```python
from build123d import *

# Parameters (mm, degrees)
SKETCH1_R                = 22
BOSS_EXTRUDE1_DEPTH      = 2.3
BOSS_EXTRUDE2_DEPTH      = 5
BOSS_EXTRUDE2_DEPTH_BACK = 21.4
SKETCH2_R                = 10.85
SKETCH3_R                = 3.9
BOSS_EXTRUDE3_DEPTH      = 9
SKETCH4_R                = 2.6
CUT_EXTRUDE1_DEPTH       = 38.761885546


with BuildPart() as part:
    # Sketch1 → Boss-Extrude1 (new body)
    with BuildSketch(Plane(origin=(0, 0, 0), x_dir=(1, 0, 0), z_dir=(0, 1, 0))):
        with Locations(Location((0, 0, 0), (0, 0, 270))):
            Circle(SKETCH1_R)
    extrude(amount=BOSS_EXTRUDE1_DEPTH)

    # Sketch2 → Boss-Extrude2 (add, two sides: drawn at the far end of the back side and taken through both)
    with BuildSketch(Plane(origin=(0, 2.3, 0), x_dir=(1, 0, 0), z_dir=(0, 1, 0)).offset(-BOSS_EXTRUDE2_DEPTH_BACK)):
        with Locations(Location((0, 0, 0), (0, 0, 270))):
            Circle(SKETCH2_R)
    extrude(amount=BOSS_EXTRUDE2_DEPTH + BOSS_EXTRUDE2_DEPTH_BACK)

    # Sketch3 → Boss-Extrude3 (add)
    with BuildSketch(Plane(origin=(0, 7.3, 0), x_dir=(1, 0, 0), z_dir=(0, 1, 0))):
        with Locations(Location((0, 0, 0), (0, 0, 270))):
            Circle(SKETCH3_R)
    extrude(amount=BOSS_EXTRUDE3_DEPTH)

    # Sketch4 → Cut-Extrude1 (cut, through all)
    with BuildSketch(Plane(origin=(0, 2.3, 0), x_dir=(1, 0, 0), z_dir=(0, 1, 0))):
        with Locations(Location((0, 17.45, 0), (0, 0, 270))):
            Circle(SKETCH4_R)
        with Locations(Location((-15.112143296, -8.725, 0), (0, 0, 270))):
            Circle(SKETCH4_R)
        with Locations(Location((15.112143296, -8.725, 0), (0, 0, 270))):
            Circle(SKETCH4_R)
    extrude(amount=-CUT_EXTRUDE1_DEPTH, mode=Mode.SUBTRACT)


solid = part.part
```
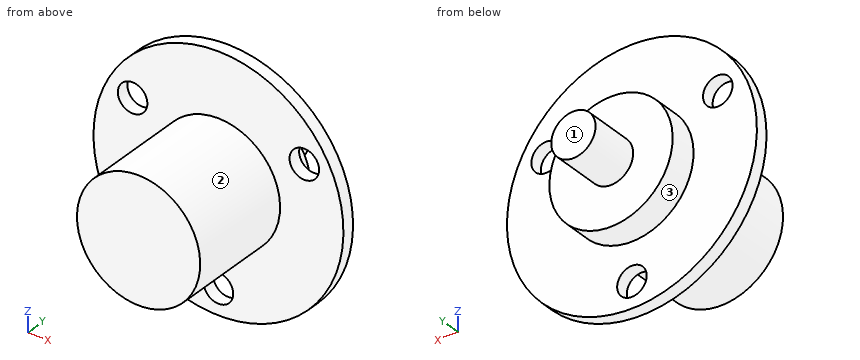
The model under review builds one solid part; all positions refer to its coordinate system, in mm. Face numbers are marked on the shaded views. A direction names the side the tool comes from. Round coordinates to 2 decimals unless told otherwise and drop trailing zeros. Write each loop counter-clockwise with the first axis right and the second up, starting at its lowest first coordinate (ties: lowest second). Pieces come first, ordered by that corner, then holes. Notation, with made-up numbers: M 0,41 L 38,41 A10 cw 38,48 Z; hole C -17.75,-3 d8. An arc over 180 degrees is marked long. Use CSV: the item, a comma, the result in double quotes. Start each with the question number.
(1) We need section C-C, the plane z = 7.5. State the section outline as (x, y) points.
(2) Clearance check with flat-ended pins moving along their axes: P1, Ø1.5, axis at x = -10.5, z = -17.5, coming from the -Y side; P2, Ø3, axis at x = 0, z = -17.45, coming from the +Y side; P3, Ø2, axis at x = 0.5, y = -5.5, coming from the +Z side; P4, Ø2, axis at y = 4.5, z = 6, coming from the +X side. State where each tip first meets the part, or that it passes through.
(3) Tool access review of the marked faces 1, 2 and 3: name each direction out of +Z, -Z, +X, -X, +Y, -Y from which nothing blocks a thin tool from reaching the whole face with its end or side.
(4) We need section B-B, the plane z = 0. State the section outline as (x, y) points.
(5) For line 1 along Y through (x, z) = (14.5, -15); line 2 along X through (y, z) = (-4.5, -0.5), list the stretches that pass through material, from the lowest coordinate up.
(6) We need section A-A, the plane x = 0. State the section outline as (y, z) points.
(7) We need section D-D, the plane y = 8.5. State the section outline as (x, z) points, then the cut area to 3 significant figures.
Findings:
1,outline,"M -20.68,0 L -17.41,0 L -17.41,2.3 L -20.68,2.3 Z; M -12.82,0 L -7.84,0 L -7.84,-19.1 L 7.84,-19.1 L 7.84,0 L 12.82,0 L 12.82,2.3 L 7.84,2.3 L 7.84,7.3 L -7.84,7.3 L -7.84,2.3 L -12.82,2.3 Z; M 17.41,0 L 20.68,0 L 20.68,2.3 L 17.41,2.3 Z"
2,P1,"y = 0"
2,P2,"through"
2,P3,"z = 10.85"
2,P4,"x = 9.63"
3,face 1,"+Z, -Z, +X, -X, +Y"
3,face 2,"-Y"
3,face 3,"+Y"
4,outline,"M -22,0 L -10.85,0 L -10.85,-19.1 L 10.85,-19.1 L 10.85,0 L 22,0 L 22,2.3 L 10.85,2.3 L 10.85,7.3 L 3.9,7.3 L 3.9,16.3 L -3.9,16.3 L -3.9,7.3 L -10.85,7.3 L -10.85,2.3 L -22,2.3 Z"
5,line 1,"0 to 2.3"
5,line 2,"-10.84 to 10.84"
6,outline,"M -19.1,-10.85 L 0,-10.85 L 0,-14.85 L 2.3,-14.85 L 2.3,-10.85 L 7.3,-10.85 L 7.3,-3.9 L 16.3,-3.9 L 16.3,3.9 L 7.3,3.9 L 7.3,10.85 L 2.3,10.85 L 2.3,22 L 0,22 L 0,10.85 L -19.1,10.85 Z; M 0,-22 L 2.3,-22 L 2.3,-20.05 L 0,-20.05 Z"
7,outline,"C 0,0 d7.8"
7,area,"47.8 mm^2"
